Autodesk Inventor part; units mm, degrees
ref_plane "YZ Plane" through (0, 0, 0) normal (1, 0, 0) x (0, 1, 0)
ref_plane "XZ Plane" through (0, 0, 0) normal (0, 1, 0) x (-1, 0, 0)
ref_plane "XY Plane" through (0, 0, 0) normal (0, 0, 1) x (1, 0, 0)
sketch "スケッチ1" plane through (0, 0, 0) normal (0, 0, 1) x (1, 0, 0)
  circle A0 centre (0, 0) radius 1.5
  dimension "d0" = 3
extrude "押し出し1" add sketch "スケッチ1" along normal blind 16
sketch "スケッチ2" plane through (0, 0, 0) normal (0, 0, -1) x (-1, 0, 0)
  circle A0 centre (0, 0) radius 2.75
  dimension "d3" = 5.5
extrude "押し出し2" add sketch "スケッチ2" along normal blind 2
fillet "フィレット1" radius 2 1 edges at (2.75, 0, -2)
thread "ねじ1"
properties part number "ネジ鍋m3,16" material "鋼、高強度、低合金"
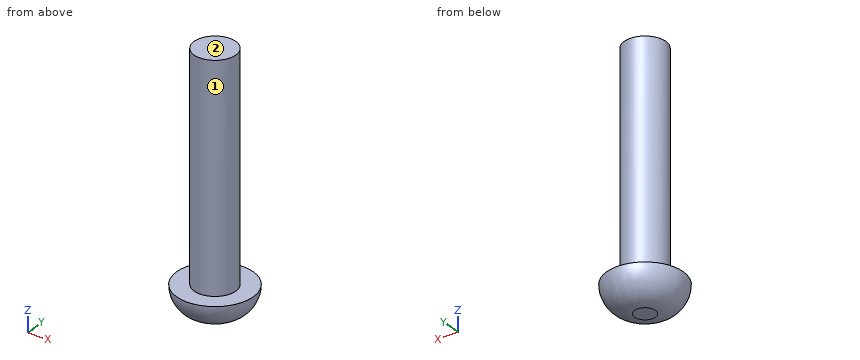
CAD build for the part. Positions are in the model's coordinates, mm. Face numbers are marked on the shaded views. A direction names the side the tool comes from. Round coordinates to 2 decimals unless told otherwise and drop trailing zeros. Loops run counter-clockwise (first coordinate to the right, second up) from the corner with the lowest first, then second, coordinate; pieces in that order, holes last. Notation, with made-up numbers: (-25, 83.5) - (12, 83.5) arc R27 cw to (12, 120.5) - close; hole circle Ø11 at (46.25, 23). An arc over 180 degrees is marked (long way). Return JSON: item names as keys, results as strings. Group by question number.
Q1. Band-saw the part on A-A on z = 5.5. Give the cut face in (x, y).
Q2. Flat gauge pins, fed straight in: pin 1 Ø1.5 at (x, y) = (1.5, -1) entering from -Z; pin 2 Ø2 at (x, y) = (-2, 0.5) entering from +Z; pin 3 Ø1 at (y, z) = (-1.5, 1.5) entering from -X. Where does each tip first touch, or does it go through?
Q3. Drill centre lines: line 1 along Y through (x, z) = (-0.1, 8); line 2 along Y through (x, z) = (1.3, 11.5); line 3 along Z through (x, y) = (-1, 1.4). Where is each one in solid material? Low to high. Write a range as [from, to].
Q4. Tool access for the marked faces 1 and 2: list every direction of +Z, -Z, +X, -X, +Y, -Y with a clear straight run to the whole face (end or side of a thin tool).
Solutions:
{
 "1": {"outline": "circle Ø3 at (0, 0)"},
 "2": {"pin 1": "stops at z = -1.98", "pin 2": "stops at z = 16", "pin 3": "stops at x = -1.12"},
 "3": {"line 1": "y = [-1.5, 1.5]", "line 2": "y = [-0.75, 0.75]", "line 3": "z = [-1.75, 0]"},
 "4": {"face 1": "+Z", "face 2": "+Z, +X, -X, +Y, -Y"}
}
